```python
from build123d import *

# Parameters (mm, degrees)
F0_R     = 14.2875
F1_DEPTH = 6.35
F2_DEPTH = 101.6


with BuildPart() as f1:
    # F0 (on Front) → F1 (new body)
    with BuildSketch(Plane.XZ):
        with BuildLine():
            Line((328.093377, -270.84429), (359.655066, -302.414026))
            ThreePointArc((359.655066, -302.414026), (0, 469.9), (-359.655066, -302.414026))
            Line((-359.655066, -302.414026), (-328.00754, -270.758432))
            ThreePointArc((-328.00754, -270.758432), (0.134045, 425.555623), (328.093377, -270.84429))
        make_face()
        with Locations((-435.780706, -117.80084)):
            Circle(F0_R, mode=Mode.SUBTRACT)
        with Locations((433.236139, -118.925363)):
            Circle(F0_R, mode=Mode.SUBTRACT)
        with Locations((-435.479391, 115.051521)):
            Circle(F0_R, mode=Mode.SUBTRACT)
        with Locations((-318.792264, 316.556925)):
            Circle(F0_R, mode=Mode.SUBTRACT)
        with Locations((-116.985546, 432.722159)):
            Circle(F0_R, mode=Mode.SUBTRACT)
        with Locations((433.537454, 113.926999)):
            Circle(F0_R, mode=Mode.SUBTRACT)
        with Locations((115.866816, 432.420844)):
            Circle(F0_R, mode=Mode.SUBTRACT)
        with Locations((317.372219, 315.733717)):
            Circle(F0_R, mode=Mode.SUBTRACT)
    extrude(amount=F1_DEPTH)

    # F0 (on Front) → F2 (join)
    with BuildSketch(Plane.XZ):
        with BuildLine():
            Line((323.581604, -266.331367), (328.093377, -270.84429))
            ThreePointArc((328.093377, -270.84429), (0.134045, 425.555623), (-328.00754, -270.758432))
            Line((-328.00754, -270.758432), (-323.495767, -266.245508))
            ThreePointArc((-323.495767, -266.245508), (0.133875, 419.208866), (323.581604, -266.331367))
        make_face()
    extrude(amount=F2_DEPTH)


solid = f1.part
```
Input: part model. Units: mm. Frame: model coordinates. Coordinates: 2 decimals unless noted, no trailing zeros. Loops run counter-clockwise (first coordinate to the right, second up) from the corner with the lowest first, then second, coordinate; pieces in that order, holes last.
Q1. Section C-C, the plane y = -72. Return the cut outline in (x, z), and give its area (3 significant figures).
Results are:
outline: (-328.01, -270.76) - (-323.5, -266.25) arc R419.1 cw (long way) to (323.58, -266.33) - (328.09, -270.84) arc R425.45 ccw (long way) to start
area: 12,100 mm2
Q2. Contact query for flat-ended pins moving along their axis: pin 1 (4 mm diameter, centred on y = -75.5, z = 320.5, fed in from +X); pin 2 (4 mm diameter, centred on y = -23.5, z = 118, fed in from +X); pin 3 (6 mm diameter, centred on x = -311.5, y = -30.5, fed in from -Z). Output: stop coordinate, or through.
Results are:
pin 1: stops at x = 282.27
pin 2: stops at x = 409.44
pin 3: stops at z = 277.03
Q3. Section A-A, the plane x = 349.5. Return the cut outline in (y, z).
Results are:
outline: (-101.6, -242.61) - (-6.35, -242.61) - (-6.35, -292.26) - (0, -292.26) - (0, -231.3) - (-101.6, -231.3) - close; (-101.6, 231.52) - (0, 231.52) - (0, 314.1) - (-6.35, 314.1) - (-6.35, 242.82) - (-101.6, 242.82) - close
Q4. Line query: line 1 along Z through (x, y) = (4, -72); line 2 along Z through (x, y) = (-329.5, -15.5); line 3 along X through (y, z) = (-56, 71). Output: solid intervals per line, ascending.
Results are:
line 1: z = 419.19 to 425.54
line 2: z = -268.94 to -258.78, 259 to 269.15
line 3: x = -419.42 to -412.98, 413.14 to 419.58
Q5. Section B-B, the plane z = -49.5. Return the cut outline in (x, y).
Results are:
outline: (-467.29, -6.35) - (-422.47, -6.35) - (-422.47, -101.6) - (-416.08, -101.6) - (-416.08, 0) - (-467.29, 0) - close; (416.23, -101.6) - (422.63, -101.6) - (422.63, -6.35) - (467.29, -6.35) - (467.29, 0) - (416.23, 0) - close
Q6. Mould query, pull axis Z, two halves, no side actions, for faces 1 (the flat face through (-2, -6.35, 429)), 2 (the cylindrical face through (-450.054, -3.131, -117.173)), 3 (the cylindrical face through (13.6, -53.31, 425.34)). Classes: +Z half, -Z half, draft (parallel to the pull), parting line (faces both ways), or undercut.
Results are:
face 1: draft
face 2: undercut
face 3: parting line
Q7. Section D-D, the plane x = 0. Return the cut outline in (y, z).
Results are:
outline: (-101.6, 419.21) - (0, 419.21) - (0, 469.9) - (-6.35, 469.9) - (-6.35, 425.56) - (-101.6, 425.56) - close
